Check sheet for the modelled part. Datum: model origin and axes. Units: mm. Round coordinates to 2 decimals unless told otherwise and drop trailing zeros. Order: outer loops, then holes, each group sorted by start corner. A loop starts at its lowest first (then second) coordinate and runs counter-clockwise, first axis right, second up. Notation, with made-up numbers: M 46.5,74.25 L 100.5,74.25 A23 cw 100.5,97.25 Z; hole C -25.75,87 d9. An arc over 180 degrees is marked long. One line per item, written item: value. Start each with the question number.
(1) Cross-section at C-C, the plane x = 25. Enter the section's corners in (y, z).
(2) Thickness scan on L1, parallel to Y at x = -50, z = 1.65; L2, parallel to Y at x = -64.5, z = 0.25; L3, parallel to Y at x = 52, z = 0.65. Record the ranges inside material, lowest first.
(3) Depth check by flat-ended pin: pin 1 Ø14.5 at (x, y) = (26.64, 29.03) entering from +Z; pin 2 Ø0.9 at (y, z) = (-15.5, 2) entering from -X. Enter the tip coordinate at first touch or a pass-through.
(4) Cross-section at A-A, the plane x = 63. Enter the section's corners in (y, z).
(5) Cross-section at B-B, the plane z = 0.65. Count the separate pieces of the cut face and the enclosed holes in it, and give its area (3 significant figures).
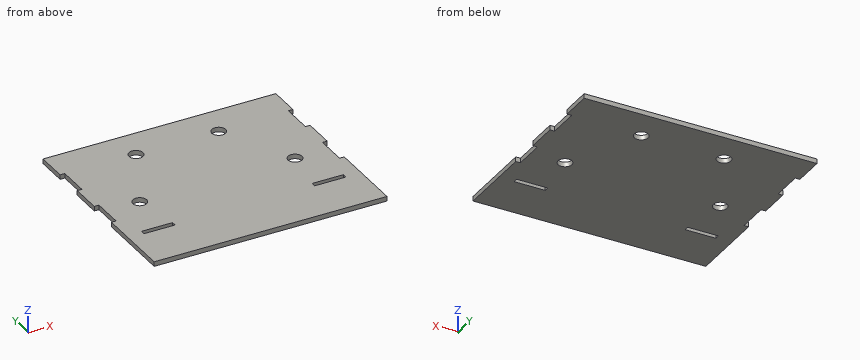
from build123d import *

# Parameters (mm, degrees)
SKETCH1_W           = 150
SKETCH1_H           = 100
BOSS_EXTRUDE1_DEPTH = 3
SKETCH2_W           = 3
SKETCH2_H           = 20
SKETCH2_W_2         = 20
SKETCH2_H_2         = 3
CUT_EXTRUDE1_DEPTH  = 3
SKETCH3_W           = 150
SKETCH3_H           = 3
BOSS_EXTRUDE2_DEPTH = 30
SKETCH5_R           = 4.5
CUT_EXTRUDE2_DEPTH  = 10
SKETCH6_R           = 4.5
CUT_EXTRUDE3_DEPTH  = 10


with BuildPart() as part:
    # Sketch1 → Boss-Extrude1 (new body)
    with BuildSketch(Plane.XY):
        Rectangle(SKETCH1_W, SKETCH1_H)
    extrude(amount=BOSS_EXTRUDE1_DEPTH)

    # Sketch2 → Cut-Extrude1 (cut)
    with BuildSketch(Plane.XY.offset(3)):
        with Locations((73.5, 20)):
            Rectangle(SKETCH2_W, SKETCH2_H)
        with Locations((73.5, -20)):
            Rectangle(SKETCH2_W, SKETCH2_H)
        with Locations((-73.5, -20)):
            Rectangle(SKETCH2_W, SKETCH2_H)
        with Locations((-73.5, 20)):
            Rectangle(SKETCH2_W, SKETCH2_H)
        with Locations((-55, -48.5)):
            Rectangle(SKETCH2_W_2, SKETCH2_H_2)
        with Locations((55, -48.5)):
            Rectangle(SKETCH2_W_2, SKETCH2_H_2)
    extrude(amount=-CUT_EXTRUDE1_DEPTH, mode=Mode.SUBTRACT)

    # Sketch3 → Boss-Extrude2 (add)
    with BuildSketch(Plane.XZ.offset(50)):
        with Locations((0, 1.5)):
            Rectangle(SKETCH3_W, SKETCH3_H)
    extrude(amount=BOSS_EXTRUDE2_DEPTH)

    # Sketch5 → Cut-Extrude2 (cut)
    with BuildSketch(Plane.XY.offset(3)):
        with Locations((50, -17.807715926)):
            Circle(SKETCH5_R)
        with Locations((-50, -17.807715926)):
            Circle(SKETCH5_R)
    extrude(amount=-CUT_EXTRUDE2_DEPTH, mode=Mode.SUBTRACT)

    # Sketch6 → Cut-Extrude3 (cut)
    with BuildSketch(Plane(origin=(0, 0, 0), x_dir=(-1, 0, 0), z_dir=(0, 0, -1))):
        with Locations((26.644067797, 29.026784983)):
            Circle(SKETCH6_R)
        with Locations((-26.644067797, 29.026784983)):
            Circle(SKETCH6_R)
    extrude(amount=-CUT_EXTRUDE3_DEPTH, mode=Mode.SUBTRACT)


solid = part.part
Values found:
1. outline: M -80,0 L 24.84,0 L 24.84,3 L -80,3 Z; M 33.22,0 L 50,0 L 50,3 L 33.22,3 Z
2. L1: -80 to -50, -47 to -22.31, -13.31 to 50
2. L2: -80 to -50, -47 to 50
2. L3: -80 to -50, -47 to -21.84, -13.78 to 50
3. pin 1: z = 3
3. pin 2: x = -72
4. outline: M -80,0 L -50,0 L -50,3 L -80,3 Z; M -47,0 L 50,0 L 50,3 L -47,3 Z
5. separate pieces: 1
5. enclosed holes: 6
5. area: 18,900 mm^2
